from build123d import *

# Parameters (mm, degrees)
EXTRUDE_3_DEPTH     = 2
EXTRUDE_3_2_DEPTH   = 2
SKETCH_2_R          = 3.75
SKETCH_2_R_2        = 2.5
EXTRUDE_5_DEPTH     = 3
EXTRUDE_START       = 2
SKETCH_3_R          = 3.75
SKETCH_3_R_2        = 2.5
EXTRUDE_6_DEPTH     = 2
SKETCH_4_R          = 0.5
CUT_EXTRUDE_1_DEPTH = 2
SKETCH_5_R          = 2.5
EXTRUDE_7_DEPTH     = 1
SKETCH_6_R          = 2.5
CUT_EXTRUDE_2_DEPTH = 0.5
SKETCH_7_R          = 1.25
CUT_EXTRUDE_3_DEPTH = 5
SKETCH4_R           = 0.7
CUT_EXTRUDE3_DEPTH  = 2
SKETCH5_R           = 0.7
CUT_EXTRUDE4_DEPTH  = 2


with BuildPart() as part:
    # Sketch 1 → Extrude 3 (new body)
    with BuildSketch(Plane.XY):
        with BuildLine():
            ThreePointArc((-2.88547071, -2.395111434), (-3.527252129, -1.273182005), (-3.75, 0))
            ThreePointArc((-3.75, 0), (-3.527252129, 1.273182005), (-2.88547071, 2.395111434))
            Line((-2.88547071, 2.395111434), (-21.986200069, 1.718255157))
            ThreePointArc((-21.986200069, 1.718255157), (-23.704455226, 0), (-21.986200069, -1.718255157))
            Line((-21.986200069, -1.718255157), (-2.88547071, -2.395111434))
        make_face()
    extrude(amount=EXTRUDE_3_DEPTH)



with BuildPart() as body_2:
    # Sketch 1 → Extrude 3 2 (new body)
    with BuildSketch(Plane.XY):
        with BuildLine():
            Line((21.986200069, 1.718255157), (2.88547071, 2.395111434))
            ThreePointArc((2.88547071, 2.395111434), (3.75, 0), (2.88547071, -2.395111434))
            Line((2.88547071, -2.395111434), (21.986200069, -1.718255157))
            ThreePointArc((21.986200069, -1.718255157), (23.704455226, 0), (21.986200069, 1.718255157))
        make_face()
    extrude(amount=EXTRUDE_3_2_DEPTH)


with BuildPart() as body_3:
    # Sketch 2 → Extrude 5 (new body)
    with BuildSketch(Plane.XY.offset(2)):
        Circle(SKETCH_2_R)
        Circle(SKETCH_2_R_2, mode=Mode.SUBTRACT)
    extrude(amount=EXTRUDE_5_DEPTH)


with BuildPart() as part_1:
    add(part.part)

    add(body_2.part)  # Extrude 6 merges body 2

    add(body_3.part)  # Extrude 6 merges body 3
    # Sketch 3 → Extrude 6 (add)
    with BuildSketch(Plane(origin=(0, 0, 2), x_dir=(-1, 0, 0), z_dir=(0, 0, -1)).offset(EXTRUDE_START)):
        with Locations(Location((0, 0, 0), (0, 0, 180))):
            Circle(SKETCH_3_R)
        with Locations(Location((0, 0, 0), (0, 0, 180))):
            Circle(SKETCH_3_R_2, mode=Mode.SUBTRACT)
    extrude(amount=-EXTRUDE_6_DEPTH)

    # Sketch 4 → Cut-Extrude 1 (cut)
    with BuildSketch(Plane(origin=(0, 0, 0), x_dir=(-1, 0, 0), z_dir=(0, 0, -1))):
        with Locations((-14.5, 0)):
            Circle(SKETCH_4_R)
        with Locations((-4.5, 0)):
            Circle(SKETCH_4_R)
        with Locations((-6.5, 0)):
            Circle(SKETCH_4_R)
        with Locations((-8.5, 0)):
            Circle(SKETCH_4_R)
        with Locations((-10.5, 0)):
            Circle(SKETCH_4_R)
        with Locations((-12.5, 0)):
            Circle(SKETCH_4_R)
        with Locations((4.5, 0)):
            Circle(SKETCH_4_R)
        with Locations((6.5, 0)):
            Circle(SKETCH_4_R)
        with Locations((8.5, 0)):
            Circle(SKETCH_4_R)
        with Locations((10.5, 0)):
            Circle(SKETCH_4_R)
        with Locations((12.5, 0)):
            Circle(SKETCH_4_R)
        with Locations((14.5, 0)):
            Circle(SKETCH_4_R)
    extrude(amount=-CUT_EXTRUDE_1_DEPTH, mode=Mode.SUBTRACT)

    # Sketch 5 → Extrude 7 (add)
    with BuildSketch(Plane(origin=(0, 0, 0), x_dir=(-1, 0, 0), z_dir=(0, 0, -1))):
        with Locations(Location((0, 0, 0), (0, 0, 180))):
            Circle(SKETCH_5_R)
    extrude(amount=-EXTRUDE_7_DEPTH)

    # Sketch 6 → Cut-Extrude 2 (cut)
    with BuildSketch(Plane(origin=(0, 0, 0), x_dir=(-1, 0, 0), z_dir=(0, 0, -1))):
        with Locations(Location((0, 0, 0), (0, 0, 180))):
            Circle(SKETCH_6_R)
    extrude(amount=-CUT_EXTRUDE_2_DEPTH, mode=Mode.SUBTRACT)

    # Sketch 7 → Cut-Extrude 3 (cut)
    with BuildSketch(Plane(origin=(0, 0, 0.5), x_dir=(-1, 0, 0), z_dir=(0, 0, -1))):
        Circle(SKETCH_7_R)
    extrude(amount=-CUT_EXTRUDE_3_DEPTH, mode=Mode.SUBTRACT)

    # Sketch4 → Cut-Extrude3 (cut)
    with BuildSketch(Plane(origin=(0, 0, 0), x_dir=(-1, 0, 0), z_dir=(0, 0, -1))):
        with Locations((21.4, 0)):
            Circle(SKETCH4_R)
    extrude(amount=-CUT_EXTRUDE3_DEPTH, mode=Mode.SUBTRACT)

    # Sketch5 → Cut-Extrude4 (cut)
    with BuildSketch(Plane(origin=(0, 0, 0), x_dir=(-1, 0, 0), z_dir=(0, 0, -1))):
        with Locations((-21.4, 0)):
            Circle(SKETCH5_R)
    extrude(amount=-CUT_EXTRUDE4_DEPTH, mode=Mode.SUBTRACT)


solid = part_1.part
Source: CAD feature listing. Evaluate the final solid. Frame: model axes, mm. A direction names the side the tool comes from. Give positions to 0.01 mm unless a question says otherwise; leave off trailing zeros. Order: outer loops, then holes, each group sorted by start corner. A loop starts at its lowest first (then second) coordinate and runs counter-clockwise, first axis right, second up. Notation, with made-up numbers: (53.5, 57.25) -> (74.5, 57.25) arc R18 ccw to (74.5, 64.25) -> close; hole circle Ø4 at (65.25, 24). An arc over 180 degrees is marked (long way). Write item = value, one per line.
Item 1: Section query A-A (x = 0). Output: boundary loops of the cut face in (y, z).
Check result:
outline = (-3.75, 0) -> (-2.5, 0) -> (-2.5, 0.5) -> (-1.25, 0.5) -> (-1.25, 1) -> (-2.5, 1) -> (-2.5, 5) -> (-3.75, 5) -> close; (1.25, 0.5) -> (2.5, 0.5) -> (2.5, 0) -> (3.75, 0) -> (3.75, 5) -> (2.5, 5) -> (2.5, 1) -> (1.25, 1) -> close
Item 2: Section query B-B (z = 1.45). State how many separate pieces and enclosed holes the cut face has, then the cut area to 3 significant figures.
Check result:
separate_pieces = 1
enclosed_holes = 15
area = 173 mm²
Item 3: Section query D-D (x = -21.4). Output: boundary loops of the cut face in (y, z), then the cut area to 3 significant figures.
Check result:
outline = (-1.74, 0) -> (-0.7, 0) -> (-0.7, 2) -> (-1.74, 2) -> close; (0.7, 0) -> (1.74, 0) -> (1.74, 2) -> (0.7, 2) -> close
area = 4.16 mm²
Item 4: Ray query, probe 1 along Y at (x, z) = (0, 0.25); probe 2 along Z at (x, y) = (-18, 0.25); probe 3 along Y at (x, z) = (-2, 2.55). Return the intervals inside material, ascending.
Check result:
probe_1 = -3.75 to -2.5, 2.5 to 3.75
probe_2 = 0 to 2
probe_3 = -3.17 to -1.5, 1.5 to 3.17
Item 5: Section query C-C (x = -14.5). Output: boundary loops of the cut face in (y, z), then the cut area to 3 significant figures.
Check result:
outline = (-1.98, 0) -> (-0.5, 0) -> (-0.5, 2) -> (-1.98, 2) -> close; (0.5, 0) -> (1.98, 0) -> (1.98, 2) -> (0.5, 2) -> close
area = 5.93 mm²
Item 6: Set-up query: faces 1 (the face through (1, -1, 0.5)), 2 (the face through (14, 0, 1)). Return all of +Z, -Z, +X, -X, +Y, -Y with unobstructed straight access to the full face (end or side cutting, diameter ignored); none if empty.
Check result:
face_1 = -Z
face_2 = +Z, -Z
Item 7: Mould query, pull axis Y, two halves, no side actions, for faces 3 (the face through (23.704, -0.038, 0.986)), 4 (the face through (-13.4, 0, 2)), 5 (the face through (-7, 0, 1)). Classes: +Y half, -Y half, draft (parallel to the pull), parting line (faces both ways), or undercut.
Check result:
face_3 = parting line
face_4 = draft
face_5 = undercut
Item 8: Contact query for flat-ended pins moving along their axis: pin 1 (3 mm diameter, centred on x = 0, y = 0, fed in from +Z); pin 2 (4 mm diameter, centred on x = -17.5, y = 0.5, fed in from +Z); pin 3 (2 mm diameter, centred on x = -21.4, y = 0, fed in from -Z). Output: stop coordinate, or through.
Check result:
pin_1 = 1
pin_2 = 2
pin_3 = 0
